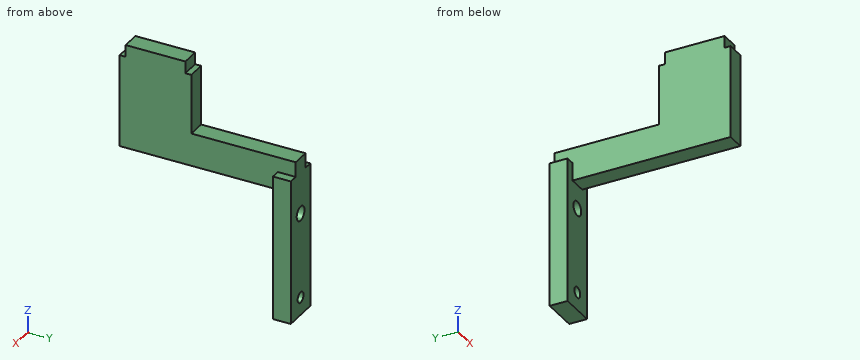
from build123d import *

# Parameters (mm, degrees)
BOSS_EXTRUDE1_START     = 7.2
SKETCH1_W               = 6
SKETCH1_H               = 3
BOSS_EXTRUDE1_DEPTH     = 24.3
BOSS_EXTRUDE2_START     = 28.5
SKETCH2_W               = 3
SKETCH2_H               = 29.475
BOSS_EXTRUDE2_DEPTH     = 17.5
CUT_EXTRUDE1_DEPTH      = 56.675089807
CUT_EXTRUDE1_DEPTH_BACK = 56.675089807
SKETCH3_R               = 1.2
SKETCH3_R_2             = 0.9
CUT_EXTRUDE2_DEPTH      = 56.675089807
CUT_EXTRUDE2_DEPTH_BACK = 56.675089807
SKETCH4_W               = 13
SKETCH4_H               = 18.475
CUT_EXTRUDE3_DEPTH      = 56.675089807
CUT_EXTRUDE3_DEPTH_BACK = 56.675089807
SKETCH5_W               = 3
SKETCH5_H               = 2.5


with BuildPart() as part:
    # Sketch1 → Boss-Extrude1 (new body)
    with BuildSketch(Plane.XY.offset(BOSS_EXTRUDE1_START)):
        with Locations((17.8, 21.975)):
            Rectangle(SKETCH1_W, SKETCH1_H)
    extrude(amount=BOSS_EXTRUDE1_DEPTH)

    # Sketch2 → Boss-Extrude2 (add)
    with BuildSketch(Plane.XY.offset(BOSS_EXTRUDE2_START)):
        with Locations((17.8, 8.7375)):
            Rectangle(SKETCH2_W, SKETCH2_H)
    extrude(amount=BOSS_EXTRUDE2_DEPTH)

    # Sketch3 → Cut-Extrude1 (cut, two sides: drawn at the far end of the back side and taken through both)
    with BuildSketch(Plane(origin=(0, 0, 0), x_dir=(1, 0, 0), z_dir=(0, 1, 0)).offset(-CUT_EXTRUDE1_DEPTH_BACK)):
        with Locations(Location((17.8, -24.5, 0), (0, 0, 270))):
            Circle(SKETCH3_R)
        with Locations(Location((17.8, -10.2, 0), (0, 0, 270))):
            Circle(SKETCH3_R_2)
    extrude(amount=CUT_EXTRUDE1_DEPTH + CUT_EXTRUDE1_DEPTH_BACK, mode=Mode.SUBTRACT)

    # Sketch4 → Cut-Extrude2 (cut, two sides: drawn at the far end of the back side and taken through both)
    with BuildSketch(Plane(origin=(0, 0, 0), x_dir=(0, 0, -1), z_dir=(1, 0, 0)).offset(-CUT_EXTRUDE2_DEPTH_BACK)):
        with Locations((-40.5, 15.2375)):
            Rectangle(SKETCH4_W, SKETCH4_H)
    extrude(amount=CUT_EXTRUDE2_DEPTH + CUT_EXTRUDE2_DEPTH_BACK, mode=Mode.SUBTRACT)

    # Sketch5 → Cut-Extrude3 (cut, two sides: drawn at the far end of the back side and taken through both)
    with BuildSketch(Plane(origin=(0, 0, 0), x_dir=(0, 0, -1), z_dir=(1, 0, 0)).offset(-CUT_EXTRUDE3_DEPTH_BACK)):
        with Locations((-45.5, -6.25)):
            Rectangle(SKETCH5_W, SKETCH5_H)
        with Locations((-45.5, 6.25)):
            Rectangle(SKETCH5_W, SKETCH5_H)
    extrude(amount=CUT_EXTRUDE3_DEPTH + CUT_EXTRUDE3_DEPTH_BACK, mode=Mode.SUBTRACT)


solid = part.part
Geometry: final body of the model. Coordinates: model frame, mm. Coordinates: 2 decimals unless noted, no trailing zeros. Order: outer loops, then holes, each group sorted by start corner. A loop starts at its lowest first (then second) coordinate and runs counter-clockwise, first axis right, second up.
(1) Section query D-D (y = 19.5). Return the cut outline in (x, z), plus the area to 3 significant figures.
(2) First-contact query: pin 1 (3 mm diameter, centred on x = 16.5, y = 15, fed in from +Z); pin 2 (6 mm diameter, centred on y = 9, z = 36, fed in from -X); pin 3 (3.5 mm diameter, centred on x = 18.5, y = 7, fed in from -Z). Flat tips, straight axial feed; report the tip coordinate or a pass-through.
(3) Section query A-A (z = 10.2). Return the cut outline in (x, y) (3 decimals), plus the area to 3 significant figures.
(4) Material intervals for probe 1 along Z at (x, y) = (17.8, 21.1); probe 2 along X at (y, z) = (22.45, 24.5); probe 3 along X at (y, z) = (22.4, 10.2), sorted ascending.
(5) Section query C-C (z = 31). Return the cut outline in (x, y) (3 decimals).
(6) Section query B-B (x = 17.8). Return the cut outline in (y, z) (3 decimals), plus the area to 3 significant figures.
Solution:
1. outline: (16.3, 28.5) - (19.3, 28.5) - (19.3, 34) - (16.3, 34) - close
1. area: 16.5 mm2
2. pin 1: stops at z = 34
2. pin 2: stops at x = 16.3
2. pin 3: stops at z = 28.5
3. outline: (14.8, 20.475) - (16.9, 20.475) - (16.9, 23.475) - (14.8, 23.475) - close; (18.7, 20.475) - (20.8, 20.475) - (20.8, 23.475) - (18.7, 23.475) - close
3. area: 12.6 mm2
4. probe 1: z = 7.2 to 9.3, 11.1 to 23.3, 25.7 to 34
4. probe 2: x = 14.8 to 16.6, 19 to 20.8
4. probe 3: x = 14.8 to 16.9, 18.7 to 20.8
5. outline: (14.8, 20.475) - (16.3, 20.475) - (16.3, -6) - (19.3, -6) - (19.3, 20.475) - (20.8, 20.475) - (20.8, 23.475) - (14.8, 23.475) - close
6. outline: (-6, 28.5) - (20.475, 28.5) - (20.475, 25.7) - (23.475, 25.7) - (23.475, 34) - (6, 34) - (6, 44) - (5, 44) - (5, 46) - (-5, 46) - (-5, 44) - (-6, 44) - close; (20.475, 7.2) - (23.475, 7.2) - (23.475, 9.3) - (20.475, 9.3) - close; (20.475, 11.1) - (23.475, 11.1) - (23.475, 23.3) - (20.475, 23.3) - close
6. area: 353 mm2
